Job drawing, mm, ordinate dimensions from the low corner. One solid piece. A direction names the side the tool comes from. Give positions to 0.01 mm unless a question says otherwise; leave off trailing zeros. Write each loop counter-clockwise with the first axis right and the second up, starting at its lowest first coordinate (ties: lowest second). Pieces come first, ordered by that corner, then holes. Notation, with made-up numbers: (44.5, 31) - (72.5, 31) arc R24 cw to (72.5, 58) - close; hole circle Ø11 at (61.25, -7). An arc over 180 degrees is marked (long way). Answer in a Markdown table with one row per item. Add a question column.
1. Band-saw the part on C-C on z = 2.5. Write the cut outline in (x, y), plus the area to 3 significant figures.
2. Band-saw the part on A-A on x = 6.5. Write the cut outline in (y, z).
3. Drop flat-ended pins along their axis: pin 1 Ø2 at (x, y) = (6, 3.5) entering from -Z; pin 2 Ø1.5 at (x, z) = (9.5, 5) entering from +Y; pin 3 Ø2 at (x, y) = (11.5, 1.5) entering from +Z; pin 4 Ø1 at (y, z) = (2.5, 3.5) entering from -X. Give the stop position or say it passes through.
4. Which spindle directions (+Z, -Z, +X, -X, +Y, -Y) get a long thin tool onto all of the face, cutting with end or side? Do the marked faces 5, 6 and 7. Say none if no direction does.
5. Band-saw the part on B-B on y = 2.1. Write the cut outline in (x, z), plus the area to 3 significant figures.
6. Pull direction Y, two halves, no side cores. Call the marked faces 1, 2, 3 and 4: released by +Y, released by -Y, zero draft, split by the parting line, or undercut.
7. Probe line 1 along Z through (x, y) = (4, 0.4); line 2 along X through (y, z) = (1.65, 3); line 3 along X through (y, z) = (2.95, 0.5). List the from-to ranges inside material, lowest first.
8. Band-saw the part on D-D on y = 0.8. Write the cut outline in (x, z).
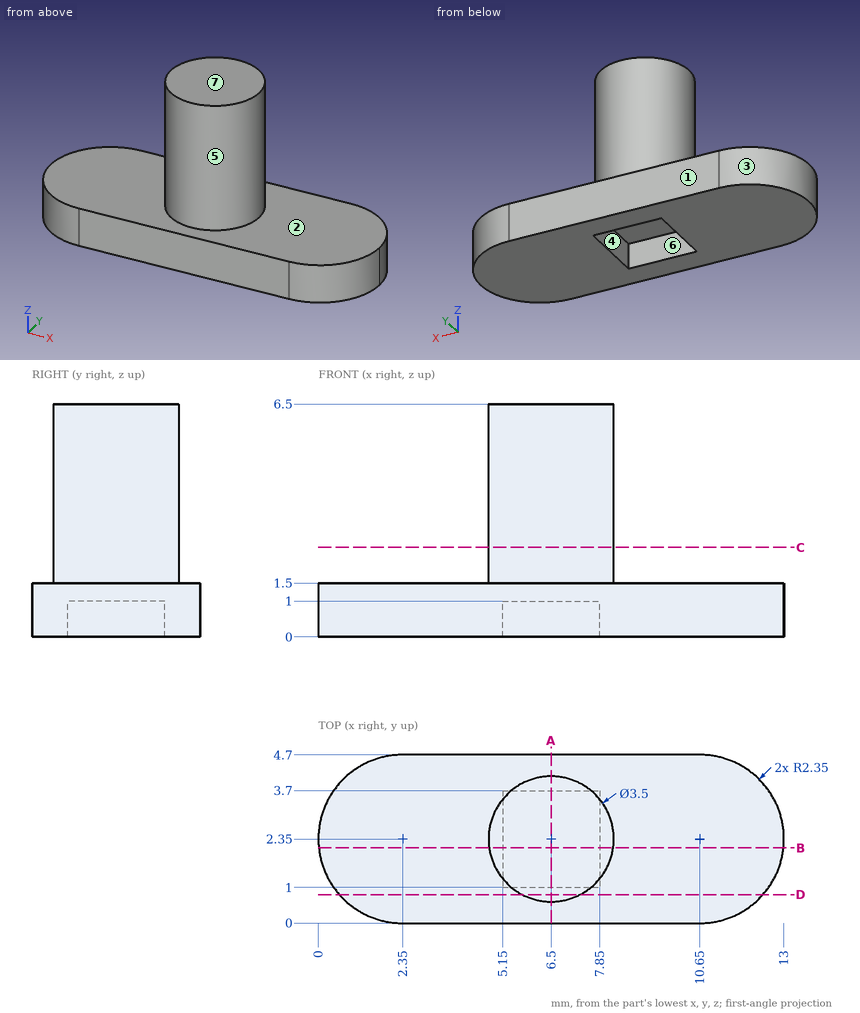
Values:
| question | item | result |
|---|---|---|
| 1 | outline | circle Ø3.5 at (6.5, 2.35) |
| 1 | area | 9.62 mm² |
| 2 | outline | (0, 0) - (1, 0) - (1, 1) - (3.7, 1) - (3.7, 0) - (4.7, 0) - (4.7, 1.5) - (4.1, 1.5) - (4.1, 6.5) - (0.6, 6.5) - (0.6, 1.5) - (0, 1.5) - close |
| 3 | pin 1 | stops at z = 0 |
| 3 | pin 2 | passes through |
| 3 | pin 3 | stops at z = 1.5 |
| 3 | pin 4 | stops at x = 4.75 |
| 4 | face 5 | +Z |
| 4 | face 6 | -Z |
| 4 | face 7 | +Z, +X, -X, +Y, -Y |
| 5 | outline | (0.01, 0) - (5.15, 0) - (5.15, 1) - (7.85, 1) - (7.85, 0) - (12.99, 0) - (12.99, 1.5) - (8.23, 1.5) - (8.23, 6.5) - (4.77, 6.5) - (4.77, 1.5) - (0.01, 1.5) - close |
| 5 | area | 34.1 mm² |
| 6 | face 1 | released by +Y |
| 6 | face 2 | zero draft |
| 6 | face 3 | split by the parting line |
| 6 | face 4 | undercut |
| 7 | line 1 | z = 0 to 1.5 |
| 7 | line 2 | x = 4.9 to 8.1 |
| 7 | line 3 | x = 0.08 to 5.15, 7.85 to 12.92 |
| 8 | outline | (0.58, 0) - (12.42, 0) - (12.42, 1.5) - (7.31, 1.5) - (7.31, 6.5) - (5.69, 6.5) - (5.69, 1.5) - (0.58, 1.5) - close |
